Could you check a few things on this model? Use its own coordinates, in mm. Face numbers are marked on the shaded views. A direction names the side the tool comes from. Give positions to 0.01 mm unless a question says otherwise; leave off trailing zeros. Order: outer loops, then holes, each group sorted by start corner. A loop starts at its lowest first (then second) coordinate and runs counter-clockwise, first axis right, second up. Notation, with made-up numbers: M 61.5,-12.5 L 72.5,-12.5 A19 ccw 72.5,8.5 Z; hole C 53.25,-25.75 d3. An arc over 180 degrees is marked long. Return JSON: item names as keys, results as strings. Group by question number.
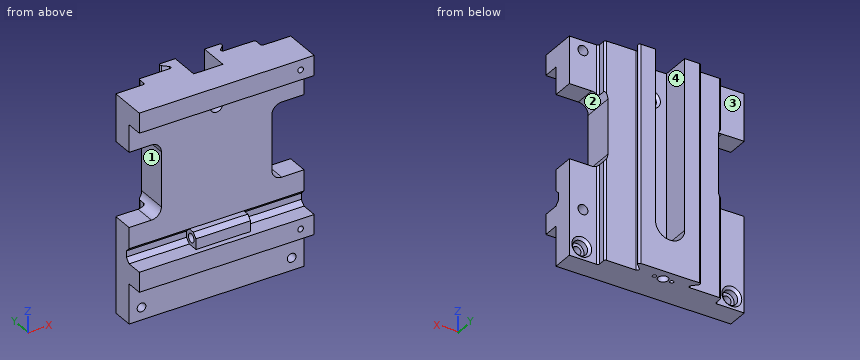
```python
from build123d import *

# Parameters (mm, degrees)
SKETCH1_R               = 4
SKETCH1_R_2             = 1.5
BOSS_EXTRUDE1_DEPTH     = 175
SKETCH2_R               = 6
CUT_EXTRUDE1_DEPTH      = 191.124958909
CUT_EXTRUDE2_DEPTH      = 191.124959013
CUT_EXTRUDE2_DEPTH_BACK = 191.124959013
SKETCH3_R               = 3.5
SKETCH3_R_2             = 5
CUT_EXTRUDE3_DEPTH      = 191.124959013
CUT_EXTRUDE3_DEPTH_BACK = 191.124959013
SKETCH4_W               = 32
SKETCH4_H               = 13
CHAMFER1_SIZE           = 2
SKETCH5_R               = 3.5
BOSS_EXTRUDE2_DEPTH     = 22
SKETCH6_R               = 4
SKETCH6_R_2             = 2.25
CUT_EXTRUDE4_DEPTH      = 18
CUT_EXTRUDE5_DEPTH      = 192.037300114
CUT_EXTRUDE5_DEPTH_BACK = 192.037300114
SKETCH6_2_R             = 2.25


with BuildPart() as part:
    # Sketch1 → Boss-Extrude1 (new body)
    with BuildSketch(Plane.XY):
        with BuildLine():
            Line((24.560660172, 20.939339828), (20.681980515, 17.060660172))
            ThreePointArc((20.681980515, 17.060660172), (20.356821388, 15.425974851), (21.742640687, 14.5))
            Line((21.742640687, 14.5), (45.5, 14.5))
            ThreePointArc((45.5, 14.5), (46.560660172, 14.060660172), (47, 13))
            Line((47, 13), (47, 8))
            ThreePointArc((47, 8), (47.439339828, 6.939339828), (48.5, 6.5))
            Line((48.5, 6.5), (70.5, 6.5))
            Line((70.5, 6.5), (70.5, -23.5))
            Line((70.5, -23.5), (-70.5, -23.5))
            Line((-70.5, -23.5), (-70.5, 6.5))
            Line((-70.5, 6.5), (-48.5, 6.5))
            ThreePointArc((-48.5, 6.5), (-47.439339828, 6.939339828), (-47, 8))
            Line((-47, 8), (-47, 13))
            ThreePointArc((-47, 13), (-46.560660172, 14.060660172), (-45.5, 14.5))
            Line((-45.5, 14.5), (-21.742640687, 14.5))
            ThreePointArc((-21.742640687, 14.5), (-20.356821388, 15.425974851), (-20.681980515, 17.060660172))
            Line((-20.681980515, 17.060660172), (-24.560660172, 20.939339828))
            ThreePointArc((-24.560660172, 20.939339828), (-24.885819299, 22.574025149), (-23.5, 23.5))
            Line((-23.5, 23.5), (23.5, 23.5))
            ThreePointArc((23.5, 23.5), (24.885819299, 22.574025149), (24.560660172, 20.939339828))
        make_face()
        with Locations((0, 14.5)):
            Circle(SKETCH1_R, mode=Mode.SUBTRACT)
        with Locations((7, 14.5)):
            Circle(SKETCH1_R_2, mode=Mode.SUBTRACT)
        with Locations((-7, 14.5)):
            Circle(SKETCH1_R_2, mode=Mode.SUBTRACT)
    extrude(amount=-BOSS_EXTRUDE1_DEPTH)

    # Sketch2 → Cut-Extrude1 (cut, through all)
    with BuildSketch(Plane(origin=(0, 0, 0), x_dir=(1, 0, 0), z_dir=(0, 1, 0))):
        with Locations(Location((-60.5, 165, 0), (0, 0, 270))):
            Circle(SKETCH2_R)
        with Locations(Location((60.5, 165, 0), (0, 0, 90))):
            Circle(SKETCH2_R)
        with BuildLine():
            Line((-11.75, 0), (-11.75, 137))
            ThreePointArc((-11.75, 137), (0, 148.75), (11.75, 137))
            Line((11.75, 137), (11.75, 0))
            ThreePointArc((11.75, 0), (0, -11.75), (-11.75, 0))
        make_face()
    extrude(amount=CUT_EXTRUDE1_DEPTH, mode=Mode.SUBTRACT)

    # Sketch3 → Cut-Extrude2 (cut, two sides: drawn at the far end of the back side and taken through both)
    with BuildSketch(Plane(origin=(0, 0, 0), x_dir=(1, 0, 0), z_dir=(0, 1, 0)).offset(-CUT_EXTRUDE2_DEPTH_BACK)):
        with Locations(Location((-60.5, 165, 0), (0, 0, 270))):
            Circle(SKETCH3_R)
        with Locations(Location((0, 24, 0), (0, 0, 270))):
            Circle(SKETCH3_R_2)
        with Locations(Location((60.5, 165, 0), (0, 0, 90))):
            Circle(SKETCH3_R)
        with BuildLine():
            Line((-70.5, 98), (-52.5, 98))
            ThreePointArc((-52.5, 98), (-46.843145751, 95.656854249), (-44.5, 90))
            Line((-44.5, 90), (-44.5, 46))
            ThreePointArc((-44.5, 46), (-46.843145751, 40.343145751), (-52.5, 38))
            Line((-52.5, 38), (-70.5, 38))
            Line((-70.5, 38), (-70.5, 98))
        make_face()
        with BuildLine():
            Line((70.5, 38), (70.5, 98))
            Line((70.5, 98), (52.5, 98))
            ThreePointArc((52.5, 98), (46.843145751, 95.656854249), (44.5, 90))
            Line((44.5, 90), (44.5, 46))
            ThreePointArc((44.5, 46), (46.843145751, 40.343145751), (52.5, 38))
            Line((52.5, 38), (70.5, 38))
        make_face()
    extrude(amount=CUT_EXTRUDE2_DEPTH + CUT_EXTRUDE2_DEPTH_BACK, mode=Mode.SUBTRACT)

    # Sketch4 → Cut-Extrude3 (cut, two sides: drawn at the far end of the back side and taken through both)
    with BuildSketch(Plane(origin=(0, 0, 0), x_dir=(0, 0, -1), z_dir=(1, 0, 0)).offset(-CUT_EXTRUDE3_DEPTH_BACK)):
        with Locations((159, -17)):
            Rectangle(SKETCH4_W, SKETCH4_H)
        Polygon((127, -23.5), (127, -10.5), (123.464466094, -6.964466094), (118.464466094, -6.964466094), (114.928932188, -10.5), (16, -10.5), (16, -23.5), align=None)
    extrude(amount=CUT_EXTRUDE3_DEPTH + CUT_EXTRUDE3_DEPTH_BACK, mode=Mode.SUBTRACT)

    # Chamfer1
    chamfer1_edges = [part.edges().sort_by_distance(p)[0] for p in [
        (0, 0, -29),
        (-60.5, 6.5, -171),
        (60.5, 6.5, -159),
    ]]
    chamfer(chamfer1_edges, length=CHAMFER1_SIZE)

    # Sketch5 → Boss-Extrude2 (add, symmetric)
    with BuildSketch(Plane(origin=(0, 0, 0), x_dir=(0, 0, -1), z_dir=(1, 0, 0))):
        Polygon((114.928932188, -15.5), (114.928932188, -10.5), (118.464466094, -6.964466094), (123.464466094, -6.964466094), (127, -10.5), (127, -19.035533906), (118.464466094, -19.035533906), align=None)
        with Locations((120.964466094, -13)):
            Circle(SKETCH5_R, mode=Mode.SUBTRACT)
    extrude(amount=BOSS_EXTRUDE2_DEPTH, both=True)

    # Sketch6 → Cut-Extrude4 (cut)
    # profile 1 of 2: a face of its own
    with BuildSketch(Plane(origin=(0, 6.5, 0), x_dir=(1, 0, 0), z_dir=(0, 1, 0))):
        with Locations(Location((59.5, 8, 0), (0, 0, 270))):
            Circle(SKETCH6_R)
        with Locations(Location((59.5, 8, 0), (0, 0, 270))):
            Circle(SKETCH6_R_2, mode=Mode.SUBTRACT)
    # profile 2 of 2: a face of its own
    with BuildSketch(Plane(origin=(0, 6.5, 0), x_dir=(1, 0, 0), z_dir=(0, 1, 0))):
        with Locations(Location((59.5, 135, 0), (0, 0, 270))):
            Circle(SKETCH6_R)
        with Locations(Location((59.5, 135, 0), (0, 0, 270))):
            Circle(SKETCH6_R_2, mode=Mode.SUBTRACT)
    extrude(amount=-CUT_EXTRUDE4_DEPTH, mode=Mode.SUBTRACT)

    # Sketch6_2 → Cut-Extrude5 (cut, two sides: drawn at the far end of the back side and taken through both)
    with BuildSketch(Plane(origin=(0, 6.5, 0), x_dir=(1, 0, 0), z_dir=(0, 1, 0)).offset(-CUT_EXTRUDE5_DEPTH_BACK)):
        with Locations(Location((59.5, 8, 0), (0, 0, 270))):
            Circle(SKETCH6_2_R)
        with Locations(Location((59.5, 135, 0), (0, 0, 270))):
            Circle(SKETCH6_2_R)
    extrude(amount=CUT_EXTRUDE5_DEPTH + CUT_EXTRUDE5_DEPTH_BACK, mode=Mode.SUBTRACT)


solid = part.part
```
1. I need wall thicknesses on L1, parallel to Z at x = -60.5, y = 1.6; L2, parallel to X at y = -6, z = -165; L3, parallel to Z at x = 59.5, y = -18.75. Which ranges of each line are inside material? Lowest first, please. Write a range as from..to.
2. Imagine slicing it at C-C, the plane y = -5. Please give me the cut outline in (x, z).
3. For pin 1 (10.5 mm diameter, centred on x = -8.5, y = -18, fed in from -Z); pin 2 (4 mm diameter, centred on x = 30.5, z = -154, fed in from -Y); pin 3 (7 mm diameter, centred on x = -29.5, z = -115, fed in from +Y); pin 4 (3.5 mm diameter, centred on y = -11.5, z = -120.5, fed in from -X), each with a flat end and sliding along its axis, tell me the tip position at first contact or that it passes through.
4. Which directions (+Z, -Z, +X, -X, +Y, -Y) give clear straight access to the entire face, cutting with the end or side of a thin tool? Please do the marked faces 1, 2, 3 and 4.
5. Imagine slicing it at D-D, the plane z = -107. Please give me the cut outline in (x, y), plus the area to 3 significant figures.
6. Imagine slicing it at A-A, the plane x = -60.5. Please give me the cut outline in (y, z).
Values:
{
 "1": {"L1": "z = -175..-171, -159..-98, -38..0", "L2": "x = -70.5..-64, -57..57, 64..70.5", "L3": "z = -143..-137.25, -132.75..-127, -16..-10.25, -5.75..0"},
 "2": {"outline": "M -70.5,-175 L 70.5,-175 L 70.5,-98 L 52.5,-98 A8 cw 44.5,-90 L 44.5,-46 A8 cw 52.5,-38 L 70.5,-38 L 70.5,0 L -70.5,0 L -70.5,-38 L -52.5,-38 A8 cw -44.5,-46 L -44.5,-90 A8 cw -52.5,-98 L -70.5,-98 Z; hole C -60.5,-165 d7; hole C 0,-24 d10; hole C 59.5,-135 d8; hole C 59.5,-8 d8; hole C 60.5,-165 d7"},
 "3": {"pin 1": "stops at z = -143", "pin 2": "stops at y = -10.5", "pin 3": "stops at y = 14.5", "pin 4": "passes through"},
 "4": {"face 1": "-X, +Y, -Y", "face 2": "+X, +Y, -Y", "face 3": "+Z, -Z, -X, +Y", "face 4": "+Z, +Y"},
 "5": {"outline": "M -70.5,-10.5 L 70.5,-10.5 L 70.5,6.5 L 48.5,6.5 A1.5 cw 47,8 L 47,13 A1.5 ccw 45.5,14.5 L 21.74,14.5 A1.5 cw 20.68,17.06 L 24.56,20.94 A1.5 ccw 23.5,23.5 L 11.75,23.5 L 11.75,0 L -11.75,0 L -11.75,23.5 L -23.5,23.5 A1.5 ccw -24.56,20.94 L -20.68,17.06 A1.5 cw -21.74,14.5 L -45.5,14.5 A1.5 ccw -47,13 L -47,8 A1.5 cw -48.5,6.5 L -70.5,6.5 Z", "area": "3,000 mm²"},
 "6": {"outline": "M -23.5,-143 L -10.5,-143 L -10.5,-161.5 L 0,-161.5 L 0,-159 L 4.5,-159 L 6.5,-157 L 6.5,-98 L -10.5,-98 L -10.5,-114.93 L -6.96,-118.46 L -6.96,-123.46 L -10.5,-127 L -23.5,-127 Z; M -23.5,-16 L -10.5,-16 L -10.5,-38 L 6.5,-38 L 6.5,0 L -23.5,0 Z; M -10.5,-175 L 6.5,-175 L 6.5,-173 L 4.5,-171 L 0,-171 L 0,-168.5 L -10.5,-168.5 Z"}
}
